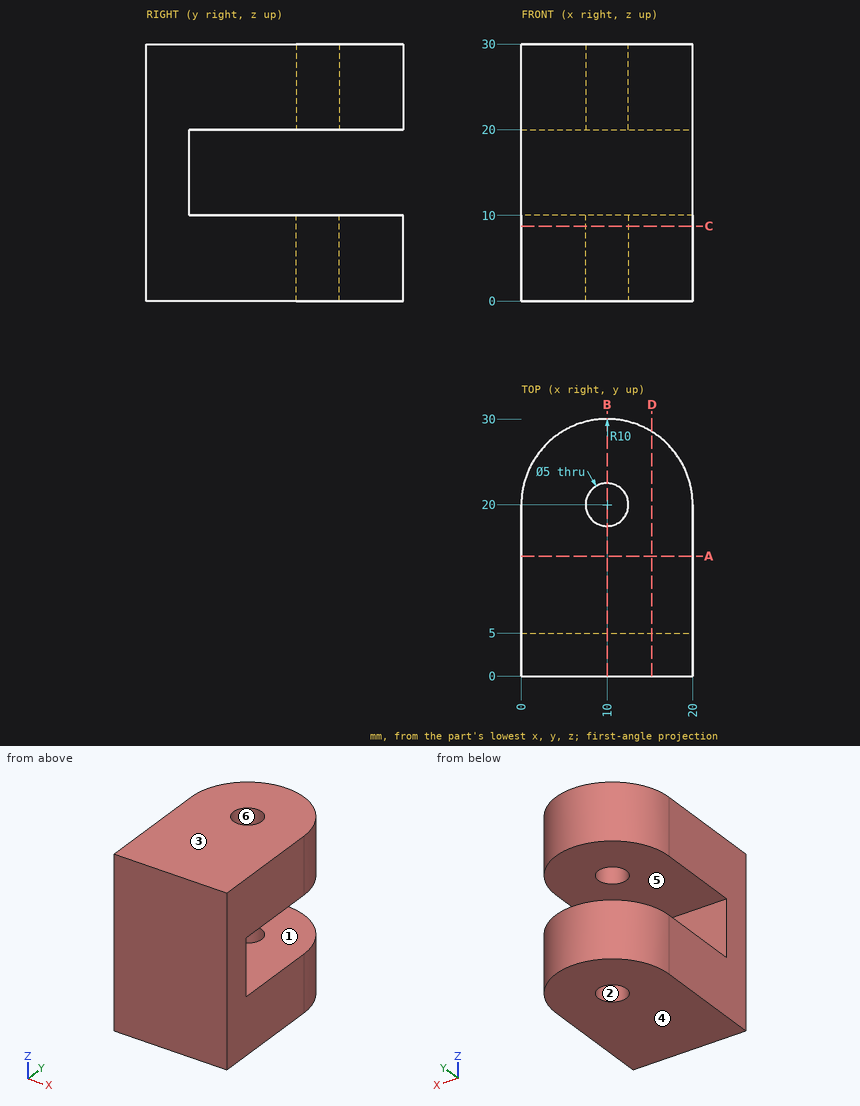
Can you work these out from the drawing? Everything is in mm from the part's minimum corner. A direction names the side the tool comes from. Coordinates: 2 decimals unless noted, no trailing zeros. Loops run counter-clockwise (first coordinate to the right, second up) from the corner with the lowest first, then second, coordinate; pieces in that order, holes last.
1. Imagine slicing it at A-A, the plane y = 14. Please give me the cut outline in (x, z), and give its area (3 significant figures).
2. For the marked faces 5 and 6, which set-ups out of +Z, -Z, +X, -X, +Y, -Y let a thin tool reach every point of the face, with its end or its side?
3. For P1, Ø3, axis at x = 10, y = 20, coming from the +Z side; P2, Ø8, axis at x = 9, z = 15, coming from the +Y side, each with a flat end and sliding along its axis, tell me the tip position at first contact or that it passes through.
4. Imagine slicing it at C-C, the plane z = 8.75. Please give me the cut outline in (x, y), and give its area (3 significant figures).
5. Imagine slicing it at D-D, the plane x = 15.25. Please give me the cut outline in (y, z), and give its area (3 significant figures).
6. Imagine slicing it at B-B, the plane x = 10. Please give me the cut outline in (y, z), and give its area (3 significant figures).
7. I need wall thicknesses on L1, parallel to Z at x = 5.5, y = 11; L2, parallel to Y at x = 10, z = 7.25; L3, parallel to X at y = 18, z = 28.25. Which ranges of each line are inside material? Lowest first, please.
8. If we mould it in two halves opening along Z, with no side actions, what happens to the marked faces 1, 2, 3 and 4? For each: pulls with the +Z half, pulls with the -Z half, needs draft (parallel to the pull), parting line crosses it, or undercut.
Taken from the geometry:
1. outline: (0, 0) - (20, 0) - (20, 10) - (0, 10) - close; (0, 20) - (20, 20) - (20, 30) - (0, 30) - close
1. area: 400 mm2
2. face 5: +X, -X, +Y
2. face 6: +Z, -Z
3. P1: passes through
3. P2: stops at y = 5
4. outline: (0, 0) - (20, 0) - (20, 20) arc R10 ccw to (0, 20) - close; hole circle Ø5 at (10, 20)
4. area: 537 mm2
5. outline: (0, 0) - (28.51, 0) - (28.51, 10) - (5, 10) - (5, 20) - (28.51, 20) - (28.51, 30) - (0, 30) - close
5. area: 620 mm2
6. outline: (0, 0) - (17.5, 0) - (17.5, 10) - (5, 10) - (5, 20) - (17.5, 20) - (17.5, 30) - (0, 30) - close; (22.5, 0) - (30, 0) - (30, 10) - (22.5, 10) - close; (22.5, 20) - (30, 20) - (30, 30) - (22.5, 30) - close
6. area: 550 mm2
7. L1: z = 0 to 10, 20 to 30
7. L2: y = 0 to 17.5, 22.5 to 30
7. L3: x = 0 to 8.5, 11.5 to 20
8. face 1: undercut
8. face 2: needs draft
8. face 3: pulls with the +Z half
8. face 4: pulls with the -Z half
